Geometry check sheet. Reference: the model listing, model coordinates, mm. Face numbers are marked on the shaded views. A direction names the side the tool comes from. Give positions to 0.01 mm unless a question says otherwise; leave off trailing zeros. Write each loop counter-clockwise with the first axis right and the second up, starting at its lowest first coordinate (ties: lowest second). Pieces come first, ordered by that corner, then holes. Notation, with made-up numbers: (24.5, -13) -> (69.5, -13) arc R21 ccw to (69.5, -1) -> close; hole circle Ø10 at (86, -35). An arc over 180 degrees is marked (long way). Write item = value, one per line. Start each with the question number.
1. Cross-section at C-C, the plane z = 28. Record the cut outline in (x, y).
2. Mould release check, pull along Y, two halves, no side actions. Record for the marked faces 4, 5, 6 and 7: pulls with the +Y half, pulls with the -Y half, needs draft (parallel to the pull), parting line crosses it, or undercut.
3. Cross-section at D-D, the plane z = 42.5. Record the cut outline in (x, y).
4. Set-up check for the marked faces 1, 2 and 3: record each of +Z, -Z, +X, -X, +Y, -Y from which the full face is reachable in a straight line by a thin tool's end or side.
5. Cross-section at B-B, the plane z = 18. Record the cut outline in (x, y), plus the area to 3 significant figures.
6. Depth check by flat-ended pin: P1, Ø15, axis at x = 14, y = 12.5, coming from the +Z side; P2, Ø6.5, axis at x = 0.5, y = 1, coming from the -Z side; P3, Ø10.5, axis at x = 0, y = 0, coming from the +Z side; P4, Ø1, axis at y = 9, z = 30.5, coming from the -X side. Enter the tip coordinate at first touch or a pass-through.
7. Thickness scan on line 1 along Y through (x, z) = (0, 1.4); line 2 along Z through (x, y) = (21.5, -38); line 3 along Z through (x, y) = (-11.5, -4.5). Record the ranges inside material, lowest first.
8. Cross-section at A-A, the plane z = 11. Record the cut outline in (x, y), plus the area to 3 significant figures.
```python
from build123d import *

# Parameters (mm, degrees)
SKETCH1_R           = 19.05
BOSS_EXTRUDE1_DEPTH = 12.7
BOSS_EXTRUDE2_DEPTH = 21.59
SKETCH4_W           = 21.59
SKETCH4_H           = 26.940768364
BOSS_EXTRUDE3_DEPTH = 43.18
CUT_EXTRUDE1_DEPTH  = 43.18
FILLET2_R           = 2.54
SKETCH6_R           = 25.4
BOSS_EXTRUDE4_DEPTH = 6.35
FILLET5_R           = 5.08
SKETCH7_R           = 4.064
CUT_EXTRUDE2_DEPTH  = 2.032


with BuildPart() as part:
    # Sketch1 → Boss-Extrude1 (new body)
    with BuildSketch(Plane.XY):
        Circle(SKETCH1_R)
    extrude(amount=BOSS_EXTRUDE1_DEPTH)

    # Sketch2 → Boss-Extrude2 (add)
    with BuildSketch(Plane.XY.offset(12.7)):
        Polygon((-19.05, 0), (0, -19.05), (19.05, 0), (0, 19.05), align=None)
    extrude(amount=BOSS_EXTRUDE2_DEPTH)

    # Sketch4 → Boss-Extrude3 (add)
    with BuildSketch(Plane(origin=(9.525, -9.525, 0), x_dir=(0, 0, -1), z_dir=(0.7071067811865477, -0.7071067811865475, 0))):
        with Locations((-23.495, 0)):
            Rectangle(SKETCH4_W, SKETCH4_H)
    extrude(amount=BOSS_EXTRUDE3_DEPTH)

    # Sketch5 → Cut-Extrude1 (cut)
    with BuildSketch(Plane(origin=(9.525, 9.525, 0), x_dir=(0, 0, -1), z_dir=(0.7071067811865475, 0.7071067811865476, 0))):
        Polygon((-34.29, -6.155864654), (-12.7, 13.470384182), (-34.29, 13.470384182), align=None)
    extrude(amount=-CUT_EXTRUDE1_DEPTH, mode=Mode.SUBTRACT)

    # Fillet2
    fillet2_edges = [part.edges().sort_by_distance(p)[0] for p in [
        (4.352853641, -4.352853641, 34.29),
    ]]
    fillet(fillet2_edges, radius=FILLET2_R)

    # Sketch6 → Boss-Extrude4 (add)
    with BuildSketch(Plane(origin=(40.057870812, -40.057870812, 0), x_dir=(0, 0, -1), z_dir=(0.7071067811865477, -0.7071067811865475, 0))):
        with Locations(Location((-23.495, 0, 0), (0, 0, 270))):
            Circle(SKETCH6_R)
    extrude(amount=BOSS_EXTRUDE4_DEPTH)

    # Fillet5
    fillet5_edges = [part.edges().sort_by_distance(p)[0] for p in [
        (40.057870812, -40.057870812, 34.29),
        (30.532870812, -49.582870812, 23.495),
        (40.057870812, -40.057870812, 12.7),
        (49.582870812, -30.532870812, 23.495),
    ]]
    fillet(fillet5_edges, radius=FILLET5_R)

    # Sketch7 → Cut-Extrude2 (cut)
    with BuildSketch(Plane(origin=(0, 0, 0), x_dir=(-1, 0, 0), z_dir=(0, 0, -1))):
        Circle(SKETCH7_R)
    extrude(amount=-CUT_EXTRUDE2_DEPTH, mode=Mode.SUBTRACT)


solid = part.part
```
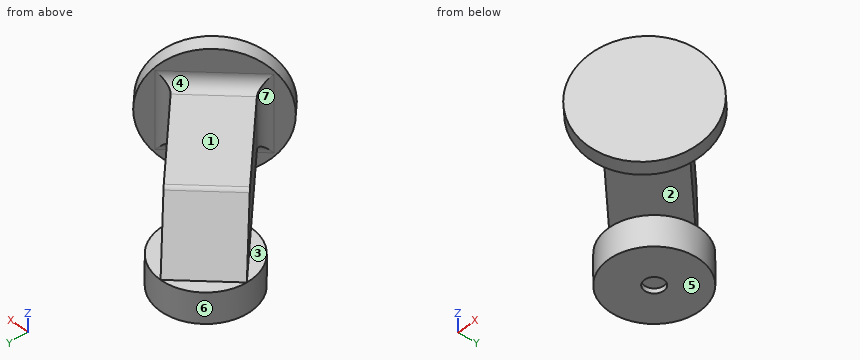
Answers:
q1.outline = (-9.22, -9.83) -> (26.94, -45.99) arc R5.08 cw to (26.94, -53.17) -> (22.38, -57.73) -> (26.87, -62.22) -> (62.22, -26.87) -> (57.73, -22.38) -> (53.17, -26.94) arc R5.08 cw to (45.99, -26.94) -> (9.83, 9.22) -> close
q2.face_4 = pulls with the +Y half
q2.face_5 = needs draft
q2.face_6 = parting line crosses it
q2.face_7 = undercut
q3.outline = (28.14, -51.97) -> (32.63, -56.46) -> (56.46, -32.63) -> (51.97, -28.14) -> close
q4.face_1 = +Z, -X, +Y
q4.face_2 = -Z
q4.face_3 = +Z, -X, -Y
q5.outline = (-15.64, -3.41) -> (26.94, -45.99) arc R5.08 cw to (26.94, -53.17) -> (22.52, -57.59) -> (27.01, -62.08) -> (62.08, -27.01) -> (57.59, -22.52) -> (53.17, -26.94) arc R5.08 cw to (45.99, -26.94) -> (3.41, 15.64) -> close
q5.area = 2,090 mm^2
q6.P1 = 34.13
q6.P2 = 0
q6.P3 = 33.29
q6.P4 = through
q7.line_1 = -19.05 to -4.06, 4.06 to 19.05
q7.line_2 = 12.7 to 34.29
q7.line_3 = 0 to 22.07
q8.outline = circle Ø38.1 at (0, 0); (24.42, -55.69) -> (28.91, -60.19) -> (60.19, -28.91) -> (55.69, -24.42) -> (53.17, -26.94) arc R5.08 cw to (49.87, -28.42) -> (28.42, -49.87) arc R5.08 cw to (26.94, -53.17) -> close
q8.area = 1,460 mm^2
